from build123d import *

# Parameters (mm, degrees)
F0_W     = 60
F0_H     = 35
F1_DEPTH = 5
F2_R     = 3.85
F3_DEPTH = 20
F4_R     = 2
F5_R     = 1.5


with BuildPart() as f1:
    # F0 (on Top) → F1 (new body)
    with BuildSketch(Plane.XY):
        Rectangle(F0_W, F0_H)
    extrude(amount=-F1_DEPTH)

    # F2 (on Top) → F3 (join)
    with BuildSketch(Plane.XY):
        with Locations((11.85, 0)):
            Circle(F2_R)
        with Locations((-11.85, 0)):
            Circle(F2_R)
    extrude(amount=F3_DEPTH)

    # F4
    f4_edges = [f1.edges().sort_by_distance(p)[0] for p in [
        (0, -17.5, 0),
        (-30, 0, 0),
        (0, 17.5, 0),
        (30, 0, 0),
        (8, 0, 20),
        (-15.7, 0, 20),
    ]]
    fillet(f4_edges, radius=F4_R)

    # F5
    f5_edges = [f1.edges().sort_by_distance(p)[0] for p in [
        (0, 17.5, -5),
        (-30, 0, -5),
        (0, -17.5, -5),
        (30, 0, -5),
    ]]
    fillet(f5_edges, radius=F5_R)


solid = f1.part
Input: part model. Units: mm. Frame: model coordinates. A direction names the side the tool comes from. Round coordinates to 2 decimals unless told otherwise and drop trailing zeros. Order: outer loops, then holes, each group sorted by start corner. A loop starts at its lowest first (then second) coordinate and runs counter-clockwise, first axis right, second up.
1. Mould query, pull axis X, two halves, no side actions, for faces 1 (the face through (29.55, 0.25, -4.57)), 2 (the face through (8, 0, 9)), 3 (the face through (0, -17.5, -3)). Classes: released by +X, released by -X, zero draft, split by the parting line, or undercut.
The answers:
face 1: released by +X
face 2: undercut
face 3: zero draft
2. Set-up query: faces 4 (the face through (-14.905, -2.343, 8.874)), 5 (the face through (0, 17.5, -3)). Return all of +Z, -Z, +X, -X, +Y, -Y with unobstructed straight access to the full face (end or side cutting, diameter ignored); none if empty.
The answers:
face 4: +Z
face 5: +Z, -Z, +X, -X, +Y
3. Cut plane C-C, the plane y = -11.5. Output: boundary loops of the cut face in (x, z), then the cut area to 3 significant figures.
The answers:
outline: (-30, -3.5) arc R1.5 ccw to (-28.5, -5) - (28.5, -5) arc R1.5 ccw to (30, -3.5) - (30, -2) arc R2 ccw to (28, 0) - (-28, 0) arc R2 ccw to (-30, -2) - close
area: 297 mm2
4. Pin query (flat end, axial travel): P1, Ø5, axis at y = 2, z = 1.5, coming from the -X side; P2, Ø6, axis at y = 1.5, z = 13, coming from the -X side. Return the tip coordinate at first contact, or that it passes through.
The answers:
P1: stops at x = -29.73
P2: stops at x = -15.7
5. Cut plane A-A, the plane x = -3.5. Output: boundary loops of the cut face in (y, z), then the cut area to 3 significant figures.
The answers:
outline: (-17.5, -3.5) arc R1.5 ccw to (-16, -5) - (16, -5) arc R1.5 ccw to (17.5, -3.5) - (17.5, -2) arc R2 ccw to (15.5, 0) - (-15.5, 0) arc R2 ccw to (-17.5, -2) - close
area: 172 mm2
6. Material intervals for line 1 (Z direction, x = 24, y = -2); line 2 (X direction, y = 1.5, z = 14.5); line 3 (X direction, y = 2.5, z = 5.5), sorted ascending.
The answers:
line 1: z = -5 to 0
line 2: x = -15.4 to -8.3, 8.3 to 15.4
line 3: x = -14.78 to -8.92, 8.92 to 14.78
7. Cut plane B-B, the plane z = 3.25. Output: boundary loops of the cut face in (x, y), then the cut area to 3 significant figures.
The answers:
outline: circle Ø7.7 at (-11.85, 0); circle Ø7.7 at (11.85, 0)
area: 93.1 mm2
